Check sheet for the modelled part. Datum: model origin and axes. Units: mm. Face numbers are marked on the shaded views. A direction names the side the tool comes from. Round coordinates to 2 decimals unless told otherwise and drop trailing zeros. Loops run counter-clockwise (first coordinate to the right, second up) from the corner with the lowest first, then second, coordinate; pieces in that order, holes last. Notation, with made-up numbers: (-2.5, 32) - (7.5, 32) arc R19 cw to (7.5, 59) - close; hole circle Ø4 at (61.5, 65). An arc over 180 degrees is marked (long way). Put each result on its own line as item: value. Start each with the question number.
```python
from build123d import *

# Parameters (mm, degrees)
SKETCH1_R               = 21
SKETCH1_R_2             = 13.5
BOSS_EXTRUDE1_DEPTH     = 18.3
BOSS_EXTRUDE3_START     = -3.175
BOSS_EXTRUDE3_DEPTH     = 3.175
SKETCH8_W               = 29.000689647
SKETCH8_H               = 11.495244731
SKETCH8_R               = 2.5875
BOSS_EXTRUDE4_DEPTH     = 3
CUT_EXTRUDE2_DEPTH      = 35.883950464
CUT_EXTRUDE2_DEPTH_BACK = 5
SKETCH7_R               = 4.9
BOSS_EXTRUDE5_START     = -18.3
SKETCH12_W              = 6
SKETCH12_H              = 8
SKETCH12_R              = 2
BOSS_EXTRUDE5_DEPTH     = 18.3001
FILLET1_R               = 2
SKETCH13_W              = 21.503284362
SKETCH13_H              = 2.04991851
SKETCH13_W_2            = 21.237930752
SKETCH13_H_2            = 2.05
CUT_EXTRUDE3_DEPTH      = 10


with BuildPart() as part:
    # Sketch1 → Boss-Extrude1 (new body)
    with BuildSketch(Plane.XY):
        Circle(SKETCH1_R)
        Circle(SKETCH1_R_2, mode=Mode.SUBTRACT)
    extrude(amount=BOSS_EXTRUDE1_DEPTH)

    # Sketch4 → Boss-Extrude3 (add)
    with BuildSketch(Plane.XY.offset(18.3).offset(BOSS_EXTRUDE3_START)):
        with BuildLine():
            Line((10.751642181, 8.164079275), (-10.751642181, 8.164079275))
            ThreePointArc((-10.751642181, 8.164079275), (-13.49956358, -0.10855024), (-10.618965376, -8.335920725))
            Line((-10.618965376, -8.335920725), (10.618965376, -8.335920725))
            ThreePointArc((10.618965376, -8.335920725), (13.49956358, -0.10855024), (10.751642181, 8.164079275))
        make_face()
    extrude(amount=BOSS_EXTRUDE3_DEPTH)

    # Sketch8 → Boss-Extrude4 (add)
    with BuildSketch(Plane.XY.offset(15.125)):
        with Locations((-0.119782029, 0.187903113)):
            Rectangle(SKETCH8_W, SKETCH8_H)
        with Locations((-0.11978203, 0.187903113)):
            Circle(SKETCH8_R, mode=Mode.SUBTRACT)
    extrude(amount=-BOSS_EXTRUDE4_DEPTH)

    # Sketch7 → Cut-Extrude2 (cut, two sides: drawn at the far end of the back side and taken through both)
    with BuildSketch(Plane.XY.offset(18.3).offset(-CUT_EXTRUDE2_DEPTH_BACK)):
        with Locations(Location((0, 0, 0), (0, 0, 180))):
            Circle(SKETCH7_R)
    extrude(amount=CUT_EXTRUDE2_DEPTH + CUT_EXTRUDE2_DEPTH_BACK, mode=Mode.SUBTRACT)

    # Sketch12 → Boss-Extrude5 (add)
    with BuildSketch(Plane.XY.offset(18.3).offset(BOSS_EXTRUDE5_START)):
        with Locations((0, 24)):
            Rectangle(SKETCH12_W, SKETCH12_H)
        with Locations((0, 24)):
            Circle(SKETCH12_R, mode=Mode.SUBTRACT)
    boss_extrude5 = extrude(amount=BOSS_EXTRUDE5_DEPTH)

    # Mirror3: Boss-Extrude5 across plane
    add(boss_extrude5.mirror(Plane.ZX))

    # Fillet1
    fillet1_edges = [part.edges().sort_by_distance(p)[0] for p in [
        (3, 28, 9.15005),
        (-3, 28, 9.15005),
        (-3, -28, 9.15005),
        (3, -28, 9.15005),
    ]]
    fillet(fillet1_edges, radius=FILLET1_R)

    # Sketch13 → Cut-Extrude3 (cut)
    with BuildSketch(Plane.XY.offset(18.3)):
        with Locations((0, 7.13912002)):
            Rectangle(SKETCH13_W, SKETCH13_H)
        with Locations((0, -7.310920725)):
            Rectangle(SKETCH13_W_2, SKETCH13_H_2)
    extrude(amount=-CUT_EXTRUDE3_DEPTH, mode=Mode.SUBTRACT)


solid = part.part
```
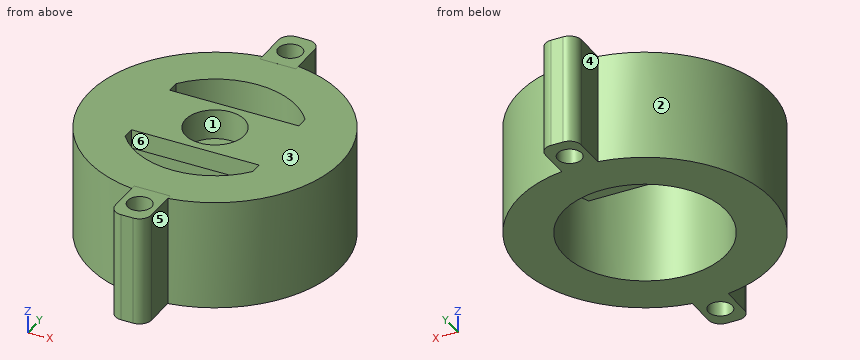
Q1. Material ranges on line 1 (Y direction, x = 0, z = 17.2); line 2 (Y direction, x = 0, z = 14.7); line 3 (Y direction, x = -2.5, z = 13.25), recorded low to high. Write a range as from..to.
Q2. Cross-section at C-C on x = 8.5. Enter the section's corners in (y, z) (3 decimals).
Q3. Cross-section at A-A on z = 17.25. Enter the section's corners in (x, y).
Q4. Cross-section at B-B on y = -24. Enter the section's corners in (x, z), and give its area (3 significant figures).
Q5. Draft check along X on the marked faces 1, 2 and 3. Enter one of: +X half, -X half, draft (parallel to the pull), parting line (faces both ways), or undercut.
Q6. Set-up check for the marked faces 4, 5 and 6: record each of +Z, -Z, +X, -X, +Y, -Y from which the full face is reachable in a straight line by a thin tool's end or side.
Q7. Cross-section at D-D on z = 7.5. Enter the section's corners in (x, y), and give its area (3 significant figures).
Q8. Depth check by flat-ended pin: pin 1 Ø11 at (x, y) = (1, 0) entering from +Z; pin 2 Ø12.5 at (x, y) = (-5.5, -2) entering from -Z (3 decimals); pin 3 Ø2 at (x, z) = (7, 2.5) entering from +Y; pin 4 Ø1.1 at (x, y) = (-1, 7.5) entering from -Z. Enter the tip coordinate at first touch or a pass-through.
Answer list:
1. line 1: y = -28..-26, -22..-13.5, -6.29..-4.9, 4.9..6.11, 13.5..22, 26..28
1. line 2: y = -28..-26, -22..-13.5, -5.56..-4.9, 4.9..5.94, 13.5..22, 26..28
1. line 3: y = -27.32..-13.27, -5.56..-0.83, 1.2..5.94, 13.27..27.32
2. outline: (-19.203, 0) - (-10.488, 0) - (-10.488, 18.3) - (-19.203, 18.3) - close; (-6.286, 15.125) - (-5.56, 15.125) - (-5.56, 12.125) - (5.936, 12.125) - (5.936, 15.125) - (6.114, 15.125) - (6.114, 18.3) - (-6.286, 18.3) - close; (10.488, 0) - (19.203, 0) - (19.203, 18.3) - (10.488, 18.3) - close
3. outline: (-3, -26) arc R2 ccw to (-1, -28) - (1, -28) arc R2 ccw to (3, -26) - (3, -20.78) arc R21 ccw to (3, 20.78) - (3, 26) arc R2 ccw to (1, 28) - (-1, 28) arc R2 ccw to (-3, 26) - (-3, 20.78) arc R21 ccw to (-3, -20.78) - close; hole (-10.75, 6.11) - (10.75, 6.11) - (10.75, 8.16) arc R13.5 ccw to (-10.75, 8.16) - close; hole (-10.62, -8.34) arc R13.5 ccw to (10.62, -8.34) - (10.62, -6.29) - (-10.62, -6.29) - close; hole circle Ø9.8 at (0, 0); hole circle Ø4 at (0, -24); hole circle Ø4 at (0, 24)
4. outline: (-3, 0) - (-2, 0) - (-2, 18.3) - (-3, 18.3) - close; (2, 0) - (3, 0) - (3, 18.3) - (2, 18.3) - close
4. area: 36.6 mm2
5. face 1: undercut
5. face 2: -X half
5. face 3: draft
6. face 4: +Z, -Z, -X, +Y
6. face 5: +Z, -Z, +X, -Y
6. face 6: +Z, -Z
7. outline: (-3, -26) arc R2 ccw to (-1, -28) - (1, -28) arc R2 ccw to (3, -26) - (3, -20.78) arc R21 ccw to (3, 20.78) - (3, 26) arc R2 ccw to (1, 28) - (-1, 28) arc R2 ccw to (-3, 26) - (-3, 20.78) arc R21 ccw to (-3, -20.78) - close; hole circle Ø27 at (0, 0); hole circle Ø4 at (0, -24); hole circle Ø4 at (0, 24)
7. area: 869 mm2
8. pin 1: stops at z = 18.3
8. pin 2: stops at z = 12.125
8. pin 3: stops at y = 20.12
8. pin 4: passes through
